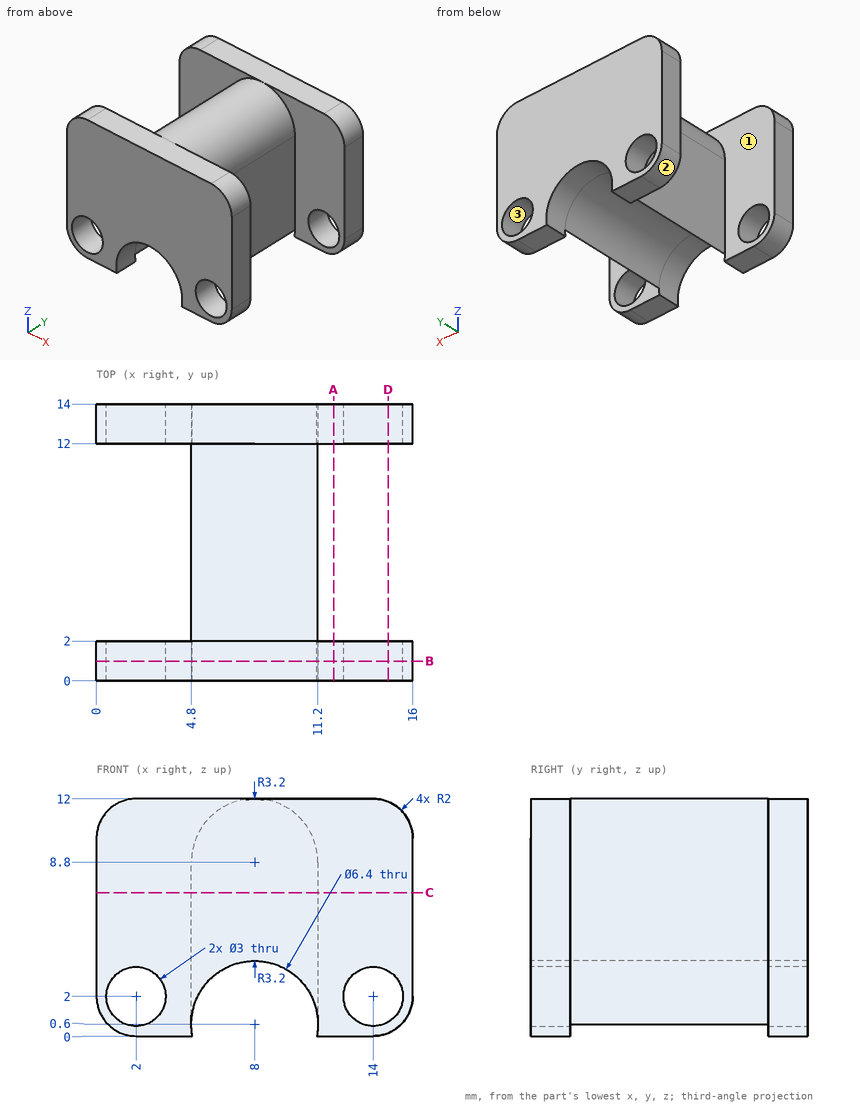
Drawing for the job (mm, zero at the part's lowest x, y, z). Coordinates: 2 decimals unless noted, no trailing zeros. Order: outer loops, then holes, each group sorted by start corner. A loop starts at its lowest first (then second) coordinate and runs counter-clockwise, first axis right, second up.
Item 1: Band-saw the part on C-C on z = 7.25. List the corners of the cut face in (x, y).
Check sheet entries:
outline: (0, 0) - (16, 0) - (16, 2) - (11.2, 2) - (11.2, 12) - (16, 12) - (16, 14) - (0, 14) - (0, 12) - (4.8, 12) - (4.8, 2) - (0, 2) - close
Item 2: Band-saw the part on D-D on x = 14.75. List the corners of the cut face in (y, z).
Check sheet entries:
outline: (0, 0.15) - (2, 0.15) - (2, 0.7) - (0, 0.7) - close; (0, 3.3) - (2, 3.3) - (2, 11.85) - (0, 11.85) - close; (12, 0.15) - (14, 0.15) - (14, 0.7) - (12, 0.7) - close; (12, 3.3) - (14, 3.3) - (14, 11.85) - (12, 11.85) - close
Item 3: Band-saw the part on A-A on x = 12. List the corners of the cut face in (y, z).
Check sheet entries:
outline: (0, 0) - (2, 0) - (2, 12) - (0, 12) - close; (12, 0) - (14, 0) - (14, 12) - (12, 12) - close
Item 4: Pin check, flat tips, straight feed: pin 1 Ø4 at (y, z) = (5.5, 6) entering from +X; pin 2 Ø1 at (y, z) = (7, 1.5) entering from -X; pin 3 Ø5 at (x, z) = (8, 0.6) entering from +Y; pin 4 Ø3 at (x, y) = (8, 3.5) entering from -Z. Stop position of each tip, or through.
Check sheet entries:
pin 1: stops at x = 11.2
pin 2: stops at x = 4.8
pin 3: passes through
pin 4: stops at z = 3.43
Item 5: Drill centre lines: L1, parallel to X at y = 0.55, z = 2; L2, parallel to Y at x = 1.25, z = 11; L3, parallel to X at y = 3, z = 8.25. Where is each one in solid material? Low to high.
Check sheet entries:
L1: x = 0 to 0.5, 3.5 to 5.12, 10.88 to 12.5, 15.5 to 16
L2: y = 0 to 2, 12 to 14
L3: x = 4.8 to 11.2
Item 6: Band-saw the part on B-B on y = 1. List the corners of the cut face in (x, z).
Check sheet entries:
outline: (0, 2) arc R2 ccw to (2, 0) - (4.86, 0) arc R3.2 cw (long way) to (11.14, 0) - (14, 0) arc R2 ccw to (16, 2) - (16, 10) arc R2 ccw to (14, 12) - (2, 12) arc R2 ccw to (0, 10) - close; hole circle Ø3 at (2, 2); hole circle Ø3 at (14, 2)
Item 7: Two-plate mould, pull along Z, no slides. Class the marked faces 1, 2 and 3: +Z half, -Z half, draft (parallel to the pull), parting line (faces both ways), or undercut.
Check sheet entries:
face 1: draft
face 2: -Z half
face 3: undercut
